Autodesk Inventor part; units mm, degrees
ref_plane "Work Plane1" through (-1520.5982, 1275.9334, 0) normal (0, 1, 0) x (0, 0, 1)
ref_plane "YZ Plane" through (0, 0, 0) normal (1, 0, 0) x (0, 1, 0)
ref_plane "XY Plane" through (0, 0, 0) normal (0, 0, 1) x (1, 0, 0)
sketch "Sketch1" plane through (0, 0, 0) normal (0, 0, 1) x (1, 0, 0)
  arc A0 (0, 2120) -> (-1624.0142, 1362.7097) centre (0, 0) ccw
  line L0 (0, 1985) -> (0, 2120)
  line L1 (0, 0) -> (2120, 0) construction
  line L2 (-1520.5982, 1275.9334) -> (-1624.0142, 1362.7097)
  line L3 (0, 0) -> (2120, 0) construction
  arc A1 (0, 1985) -> (-1520.5982, 1275.9334) centre (0, 0) ccw
  dimension "d0" = 4240
  dimension "d1" = 90
  dimension "d2" = 140
  dimension "d5" = 1985
extrude "Extrusion1" add sketch "Sketch1" along normal blind 1650
ref_plane "Work Plane1" through (-1520.5982, 1275.9334, 0) normal (0, 1, 0) x (0, 0, 1)
fillet "Fillet1" radius 15 1 edges at (-1624.0142, 1362.7097, 825)
shell "Shell2" thickness 4 removed faces 1 at (0, 2030, 550)
properties part number "Water Tank" material "Polycarbonate, Clear"
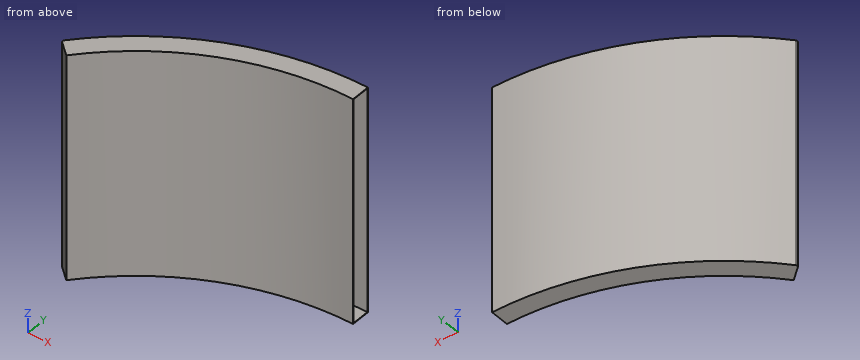
Work out the finished part from the listing and answer in its coordinate system (mm). Round coordinates to 2 decimals unless told otherwise and drop trailing zeros. Loops run counter-clockwise (first coordinate to the right, second up) from the corner with the lowest first, then second, coordinate; pieces in that order, holes last. Notation, with made-up numbers: (-30, 4) - (-6, 4) arc R7 cw to (-6, 14) - close; hole circle Ø4 at (-33.5, 80). An arc over 180 degrees is marked (long way). Use one line per item in the form item = value. Start each with the question number.
(1) Consider line 1 (Z direction, x = -1034, y = 1770); line 2 (X direction, y = 1570.5, z = 1166.5); line 3 (X direction, y = 1559.5, z = 477). Determine where each line is inside the solid, lowest interval first.
(2) Flat-ended cylindrical pins translate along their axes: P1, Ø6, axis at x = -609.5, z = 980, coming from the -Y side; P2, Ø4, axis at x = -1290.5, z = 892.5, coming from the +Y side; P3, Ø6, axis at x = -937.5, z = 1191, coming from the -Y side. Find the tip coordinate at first contact, or state that the pin passes through.
(3) Find section A-A on z = 977.5. Determine the outline of the cut face in (x, y).
Answer list:
q1.line_1 = 0 to 4, 1646 to 1650
q1.line_2 = -1424.05 to -1418.09, -1220.51 to -1213.98
q1.line_3 = -1436.09 to -1430.18, -1234.54 to -1228.08
q2.P1 = 1888.14
q2.P2 = 1683.5
q2.P3 = 1748.05
q3.outline = (-1614.26, 1374.25) arc R15 ccw to (-1612.48, 1353.03) - (-1520.6, 1275.93) arc R1985 cw to (0, 1985) - (0, 1989) arc R1989 ccw to (-1521.09, 1281.57) - (-1609.91, 1356.1) arc R11 cw to (-1611.22, 1371.65) arc R2116 cw to (0, 2116) - (0, 2120) arc R2120 ccw to start
